```python
from build123d import *

# Parameters (mm, degrees)
F0_R     = 28.575
F1_DEPTH = 40.2336
F2_R     = 10.16
F3_DEPTH = 15.7734
F4_R     = 3.302


with BuildPart() as f1:
    # F0 (on Top) → F1 (new body)
    with BuildSketch(Plane.XY):
        Circle(F0_R)
        with BuildLine():
            ThreePointArc((13.4603984155, -4.790650347), (-14.2875, 0), (13.4603984155, 4.790650347))
            Line((13.4603984155, 4.790650347), (18.5293, 4.790650347))
            Line((18.5293, 4.790650347), (18.5293, 0.035349653))
            Line((18.5293, 0.035349653), (18.5293, -0.035349653))
            Line((18.5293, -0.035349653), (18.5293, -4.790650347))
            Line((18.5293, -4.790650347), (13.4603984155, -4.790650347))
        make_face(mode=Mode.SUBTRACT)
    extrude(amount=F1_DEPTH)

    # F2 (on Top) → F3 (join)
    with BuildSketch(Plane.XY):
        with BuildLine():
            Line((5.0426470588, -28.1265414802), (57.3367647059, -18.7510276535))
            ThreePointArc((57.3367647059, -18.7510276535), (73.025, 0), (57.3367647059, 18.7510276535))
            Line((57.3367647059, 18.7510276535), (5.0426470588, 28.1265414802))
            ThreePointArc((5.0426470588, 28.1265414802), (21.9160245563, 18.3362616868), (28.575, 0))
            ThreePointArc((28.575, 0), (21.9160245563, -18.3362616868), (5.0426470588, -28.1265414802))
        make_face()
        with Locations((53.975, 0)):
            Circle(F2_R, mode=Mode.SUBTRACT)
    extrude(amount=F3_DEPTH)

    # F4
    f4_edges = [f1.edges().sort_by_distance(p)[0] for p in [
        (-28.575, 0, 40.2336),
    ]]
    fillet(f4_edges, radius=F4_R)


solid = f1.part
```
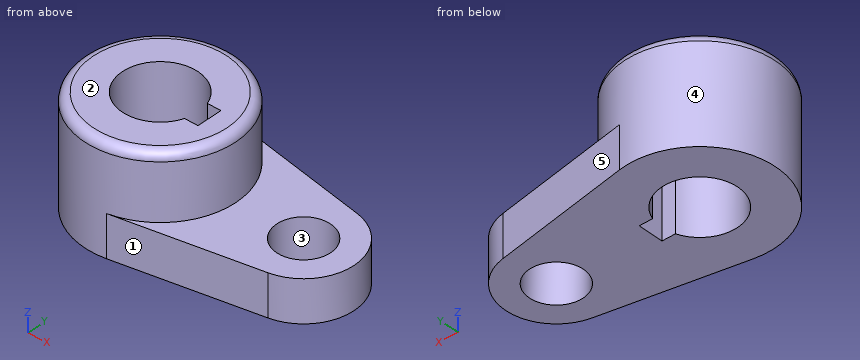
The listing builds one solid part. Answer for the finished solid, in the listing's coordinates (mm). Face numbers are marked on the shaded views. A direction names the side the tool comes from. Round coordinates to 2 decimals unless told otherwise and drop trailing zeros. Write each loop counter-clockwise with the first axis right and the second up, starting at its lowest first coordinate (ties: lowest second). Pieces come first, ordered by that corner, then holes. Notation, with made-up numbers: (-1.75, -23) -> (47.25, -23) arc R23 cw to (47.25, -4) -> close; hole circle Ø11 at (32.5, 2). An arc over 180 degrees is marked (long way). Answer as a JSON object with one key per item and string values. Group by question number.
Q1. Section A-A (x = 0) is taken. Write down the section's boundary in (y, z) (1 decimal), plus the area to 3 significant figures.
Q2. Straight lines are drawn through the part: line 1 along Y through (x, z) = (0, 11) (1 decimal); line 2 along X through (y, z) = (0, 28) (1 decimal); line 3 along Z through (x, y) = (43, -2). For each, find the intervals that lie inside material, in ascending order.
Q3. Section C-C (y = 0) is taken. Write down the section's boundary in (x, z) (1 decimal).
Q4. Determine the mould class of the marked faces 1, 2 and 3 for opening direction Y: pulls with the +Y half, pulls with the -Y half, needs draft (parallel to the pull), parting line crosses it, or undercut.
Q5. Each of these flat-tipped pins is pushed along its axis until it touches: pin 1 Ø5 at (x, z) = (-10.5, 15.5) entering from -Y; pin 2 Ø1.5 at (y, z) = (7.5, 5.5) entering from -X; pin 3 Ø5 at (x, z) = (3.5, 26.5) entering from -Y. Where does it stop, or does it pass through?
Q6. Section B-B (z = 14.5) is taken. Count the separate pieces of the cut face and the enclosed holes in it, plus the area to 3 significant figures.
Q7. Which of the six approach directions +Z, -Z, +X, -X, +Y, -Y give full straight-line access (tool end or side, diameter ignored) to the marked faces 4 and 5?
Check values:
{
 "1": {"outline": "(-28.6, 0) -> (-14.3, 0) -> (-14.3, 40.2) -> (-25.3, 40.2) arc R3.3 ccw to (-28.6, 36.9) -> close; (14.3, 0) -> (28.6, 0) -> (28.6, 36.9) arc R3.3 ccw to (25.3, 40.2) -> (14.3, 40.2) -> close", "area": "1,140 mm^2"},
 "2": {"line 1": "-28.6 to -14.3, 14.3 to 28.6", "line 2": "-28.6 to -14.3, 18.5 to 28.6", "line 3": "0 to 15.77"},
 "3": {"outline": "(-28.6, 0) -> (-14.3, 0) -> (-14.3, 40.2) -> (-25.3, 40.2) arc R3.3 ccw to (-28.6, 36.9) -> close; (18.5, 0) -> (43.8, 0) -> (43.8, 15.8) -> (28.6, 15.8) -> (28.6, 36.9) arc R3.3 ccw to (25.3, 40.2) -> (18.5, 40.2) -> close; (64.1, 0) -> (73, 0) -> (73, 15.8) -> (64.1, 15.8) -> close"},
 "4": {"face 1": "pulls with the -Y half", "face 2": "needs draft", "face 3": "undercut"},
 "5": {"pin 1": "y = -27.43", "pin 2": "x = -27.77", "pin 3": "y = -28.56"},
 "6": {"separate pieces": "1", "enclosed holes": "2", "area": "3,450 mm^2"},
 "7": {"face 4": "+Z", "face 5": "+Z, -Z, +X, +Y"}
}
